Geometry check sheet. Reference: the model listing, model coordinates, mm. A direction names the side the tool comes from. Round coordinates to 2 decimals unless told otherwise and drop trailing zeros. Loops run counter-clockwise (first coordinate to the right, second up) from the corner with the lowest first, then second, coordinate; pieces in that order, holes last. Notation, with made-up numbers: (34, 29.5) -> (41, 29.5) arc R25 cw to (41, 61.5) -> close; hole circle Ø4 at (4.25, 69). An arc over 180 degrees is marked (long way). Use one line per item in the form item = value.
from build123d import *

# Parameters (mm, degrees)
FILLET1_R = 2


with BuildPart() as part:
    # Sketch1 → Revolve1 (revolve)
    with BuildSketch(Plane.XY, mode=Mode.PRIVATE) as revolve1_sk:
        Polygon((-12.5, 1), (-12.5, -1), (-11, -1), (-11, -0.3), (-7, -0.3), (-7, -1), (-4.25, -1), (-4.25, 0.3), (-6, 0.3), (-6, 1), align=None)
    revolve(revolve1_sk.sketch.rotate(Axis((0, 0.3, 0), (0, -1, 0)), 270), axis=Axis((0, 0.3, 0), (0, -1, 0)))

    # Fillet1
    # the kernel refuses this fillet: 2 mm, written as the material it adds along each edge
    with BuildSketch(Plane(origin=(0, -0.3, 0), x_dir=(0, 0, 1), z_dir=(1, 0, 0))) as fillet1_piece_1:
        with BuildLine():
            CenterArc((8.519868415, 2), FILLET1_R, 220.541601874, 49.458398126)
            Line((7, 0.7), (6.969602632, 0.674))
            ThreePointArc((6.969602632, 0.674), (6.96, 0.35), (6.96, 0))
            Line((6.96, 0), (7, -0.04))
            Line((7, -0.04), (8.519868415, -0.04))
            Line((8.519868415, -0.04), (8.519868415, 0))
        make_face()
    revolve(axis=Axis((0, -0.3, 0), (0, -1, 0)))
    with BuildSketch(Plane(origin=(0, -0.3, 0), x_dir=(0, 0, 1), z_dir=(1, 0, 0))) as fillet1_piece_2:
        with BuildLine():
            CenterArc((9.480131585, 2), FILLET1_R, 270, 49.458398126)
            Line((9.480131585, 0), (9.480131585, -0.04))
            Line((9.480131585, -0.04), (11, -0.04))
            Line((11, -0.04), (11.04, 0))
            ThreePointArc((11.04, 0), (11.04, 0.35), (11.030397368, 0.674))
            Line((11.030397368, 0.674), (11, 0.7))
        make_face()
    revolve(axis=Axis((0, -0.3, 0), (0, -1, 0)))
    # the kernel refuses this fillet: 2 mm, written as the material it takes off along each edge
    with BuildSketch(Plane(origin=(0, 1, 0), x_dir=(0, 0, 1), z_dir=(1, 0, 0))) as fillet1_2_piece_1:
        with BuildLine():
            CenterArc((12.5 - FILLET1_R, FILLET1_R), FILLET1_R, 270, 90)
            Line((12.5 - FILLET1_R, 0), (12.5 - FILLET1_R, -FILLET1_R * 0.02))
            Line((12.5 - FILLET1_R, -FILLET1_R * 0.02), (12.5 + FILLET1_R * 0.02, -FILLET1_R * 0.02))
            Line((12.5 + FILLET1_R * 0.02, -FILLET1_R * 0.02), (12.5 + FILLET1_R * 0.02, FILLET1_R))
            Line((12.5 + FILLET1_R * 0.02, FILLET1_R), (12.5, FILLET1_R))
        make_face()
    revolve(axis=Axis((0, 1, 0), (0, -1, 0)), mode=Mode.SUBTRACT)
    with BuildSketch(Plane(origin=(0, 1, 0), x_dir=(0, 0, 1), z_dir=(1, 0, 0))) as fillet1_2_piece_2:
        with BuildLine():
            CenterArc((7.519868415, 2), FILLET1_R, 220.541601874, 49.458398126)
            Line((6, 0.7), (5.969602632, 0.674))
            ThreePointArc((5.969602632, 0.674), (5.96, 0.35), (5.96, 0))
            Line((5.96, 0), (6, -0.04))
            Line((6, -0.04), (7.519868415, -0.04))
            Line((7.519868415, -0.04), (7.519868415, 0))
        make_face()
    revolve(axis=Axis((0, 1, 0), (0, -1, 0)), mode=Mode.SUBTRACT)


solid = part.part
1. Gauge pin test, flat ends, axial feed: pin 1 (6 mm diameter, centred on x = -0.5, z = 4, fed in from +Y); pin 2 (3.5 mm diameter, centred on x = -1.5, z = -1.5, fed in from +Y). Record the tip position at first contact, or that the pin passes through.
Return value:
pin_1 = 0.94
pin_2 = through
2. Section check A-A (z = 0). Record the boundary of the cut face in (x, y), then the cut area to 3 significant figures.
Return value:
outline = (-12.5, -1) -> (-11, -1) arc R2 cw to (-9.48, -0.3) -> (-8.52, -0.3) arc R2 cw to (-7, -1) -> (-4.25, -1) -> (-4.25, 0.3) -> (-6, 0.3) arc R2 ccw to (-7.52, 1) -> (-10.5, 1) arc R2 ccw to start; (4.25, -1) -> (7, -1) arc R2 cw to (8.52, -0.3) -> (9.48, -0.3) arc R2 cw to (11, -1) -> (12.5, -1) arc R2 ccw to (10.5, 1) -> (7.52, 1) arc R2 ccw to (6, 0.3) -> (4.25, 0.3) -> close
area = 23.9 mm2
3. Mould release check, pull along Z, two halves, no side actions. Record for faces 3 (the flat face through (7, 1, -5)), 4 (the flat face through (4, 0.3, -3)): released by +Z, released by -Z, zero draft, split by the parting line, or undercut.
Return value:
face_3 = zero draft
face_4 = undercut
4. Section check B-B (x = 0). Record the boundary of the cut face in (y, z).
Return value:
outline = (-1, -12.5) arc R2 ccw to (1, -10.5) -> (1, -7.52) arc R2 ccw to (0.3, -6) -> (0.3, -4.25) -> (-1, -4.25) -> (-1, -7) arc R2 cw to (-0.3, -8.52) -> (-0.3, -9.48) arc R2 cw to (-1, -11) -> close; (-1, 4.25) -> (0.3, 4.25) -> (0.3, 6) arc R2 ccw to (1, 7.52) -> (1, 10.5) arc R2 ccw to (-1, 12.5) -> (-1, 11) arc R2 cw to (-0.3, 9.48) -> (-0.3, 8.52) arc R2 cw to (-1, 7) -> close
5. Section check D-D (y = 0.7). Record the boundary of the cut face in (x, z).
Return value:
outline = circle Ø23.11 at (0, 0); hole circle Ø12.93 at (0, 0)
6. Material ranges on line 1 along X through (y, z) = (-0.15, 0); line 2 along Z through (x, y) = (3, 0.55); line 3 along X through (y, z) = (-0.2, -3.75), recorded low to high.
Return value:
line_1 = -12.31 to -4.25, 4.25 to 12.31
line_2 = -11.37 to -5.49, 5.49 to 11.37
line_3 = -11.75 to -2, 2 to 11.75
7. Tool access check on faces 1 (the flat face through (5, -1, 0)), 2 (the flat face through (-4, -0.3, -8)). Record the directions out of +Z, -Z, +X, -X, +Y, -Y that give a thin tool (end or side, any length) a straight path to the whole face; none if there is none.
Return value:
face_1 = +Z, -Z, +X, -X, -Y
face_2 = -Y
8. Section check C-C (y = -0.65). Record the boundary of the cut face in (x, z), then the cut area to 3 significant figures.
Return value:
outline = circle Ø24.94 at (0, 0); circle Ø14.78 at (0, 0); hole circle Ø21.22 at (0, 0); hole circle Ø8.5 at (0, 0)
area = 250 mm2
